from build123d import *

# Parameters (mm, degrees)
F0_R     = 2.5
F1_DEPTH = 9.7
F2_SIZE  = 5
F3_R     = 2


with BuildPart() as f1:
    # F0 (on Top) → F1 (new body)
    with BuildSketch(Plane.XY):
        Polygon((-20, 10.480181), (-20, -20), (-10, -20), (0, -20), (20, -20), (20, 20), (10, 20), (-10, 20), (-20, 20), align=None)
        with Locations((-10, -10)):
            Circle(F0_R, mode=Mode.SUBTRACT)
        with Locations((10, -10)):
            Circle(F0_R, mode=Mode.SUBTRACT)
        with Locations((-10, 10.480181)):
            Circle(F0_R, mode=Mode.SUBTRACT)
        with Locations((10, 10.480181)):
            Circle(F0_R, mode=Mode.SUBTRACT)
    extrude(amount=F1_DEPTH)

    # F2
    f2_edges = [f1.edges().sort_by_distance(p)[0] for p in [
        (-12.5, 10.480181, 9.7),
        (7.5, 10.480181, 9.7),
        (7.5, -10, 9.7),
        (-12.5, -10, 9.7),
    ]]
    chamfer(f2_edges, length=F2_SIZE)

    # F3
    f3_edges = [f1.edges().sort_by_distance(p)[0] for p in [
        (0, -20, 9.7),
        (20, 0, 9.7),
        (0, 20, 9.7),
        (-20, 0, 9.7),
    ]]
    fillet(f3_edges, radius=F3_R)


solid = f1.part
Geometry: final body of the model. Coordinates: model frame, mm. Coordinates: 2 decimals unless noted, no trailing zeros. Loops run counter-clockwise (first coordinate to the right, second up) from the corner with the lowest first, then second, coordinate; pieces in that order, holes last. Notation, with made-up numbers: M -4.5,29 L 49.5,29 A24 cw 49.5,48 Z; hole C 39.25,-26.5 d8. An arc over 180 degrees is marked long. One line per item, written item: value. Start each with the question number.
1) Draft query along X for faces 1 (the flat face through (0, -20, 4)), 2 (the cylindrical face through (-19.4, -0.28, 9.13)), 3 (the cylindrical face through (9.46, -12.44, 2.32)). Return one class per face: released by +X, released by -X, zero draft, split by the parting line, or undercut.
2) Cut plane D-D (z = 6.75). Return loops of the section in (x, y).
3) Pin query (flat end, axial travel): P1, Ø1, axis at y = -13.5, z = 8.5, coming from the -X side; P2, Ø4, axis at y = 12.5, z = 8, coming from the +X side; P3, Ø8, axis at x = -10, y = 10.48, coming from the +Z side. Return the tip coordinate at first contact, or that it passes through.
4) Cut plane B-B (x = -10). Count the separate pieces of the cut face and the enclosed holes in it, then the cut area to 3 significant figures.
5) Material intervals for L1, parallel to Y at x = -10, z = 3.55; L2, parallel to X at y = -11.5, z = 3; L3, parallel to Y at x = 12.5, z = 5.5, sorted ascending. Write a range as from..to.
6) Cut plane C-C (z = 1). Return loops of the section in (x, y), then the cut area to 3 significant figures.
7) Cut plane A-A (y = -10). Return loops of the section in (x, z).
Evaluation:
1. face 1: zero draft
1. face 2: released by -X
1. face 3: undercut
2. outline: M -20,-20 L 20,-20 L 20,20 L -20,20 Z; hole C -10,-10 d9.1; hole C -10,10.48 d9.1; hole C 10,-10 d9.1; hole C 10,10.48 d9.1
3. P1: x = -19.98
3. P2: x = 20
3. P3: z = 6.2
4. separate pieces: 3
4. enclosed holes: 0
4. area: 239 mm^2
5. L1: -20..-12.5, -7.5..7.98, 12.98..20
5. L2: -20..-12, -8..8, 12..20
5. L3: -20..-12.15, -7.85..8.33, 12.63..20
6. outline: M -20,-20 L 20,-20 L 20,20 L -20,20 Z; hole C -10,-10 d5; hole C -10,10.48 d5; hole C 10,-10 d5; hole C 10,10.48 d5
6. area: 1,520 mm^2
7. outline: M -20,0 L -12.5,0 L -12.5,4.7 L -17.5,9.7 L -18,9.7 A2 ccw -20,7.7 Z; M -7.5,0 L 7.5,0 L 7.5,4.7 L 2.5,9.7 L -2.5,9.7 L -7.5,4.7 Z; M 12.5,0 L 20,0 L 20,7.7 A2 ccw 18,9.7 L 17.5,9.7 L 12.5,4.7 Z
